Source: CAD feature listing. Evaluate the final solid. Frame: model axes, mm. A direction names the side the tool comes from. Give positions to 0.01 mm unless a question says otherwise; leave off trailing zeros. Order: outer loops, then holes, each group sorted by start corner. A loop starts at its lowest first (then second) coordinate and runs counter-clockwise, first axis right, second up. Notation, with made-up numbers: M -36.75,59.5 L 9.25,59.5 A11 cw 9.25,79.5 Z; hole C 12.25,3.5 d3. An arc over 180 degrees is marked long. Answer as a JSON object with one key per item and string values. Group by question number.
1. Pin query (flat end, axial travel): P1, Ø3, axis at y = -12.5, z = -70.5, coming from the -X side; P2, Ø2, axis at y = -6.5, z = -92.5, coming from the -X side; P3, Ø3, axis at x = -96.5, z = -151.5, coming from the -Y side; P4, Ø20.5, axis at x = -29.5, z = -95.5, coming from the +Y side. Return the tip coordinate at first contact, or that it passes through.
2. Section query D-D (z = -73.5). Output: boundary loops of the cut face in (x, y), plus the area to 3 significant figures.
3. Section query A-A (x = -30.5). Output: boundary loops of the cut face in (y, z).
4. Material intervals for L1, parallel to X at y = -12.75, z = -97; L2, parallel to Y at x = -33.5, z = -73.5; L3, parallel to Y at x = -93.5, z = -63, sorted ascending. Write a range as [from, to].
5. Set-up query: faces 5 (the flat face through (-36, 3, -221.069)), 6 (the flat face through (-36, -9, -118.199)), 7 (the flat face through (-97, 1.27, -136)), 8 (the flat face through (28, 0, -138)). Return all of +Z, -Z, +X, -X, +Y, -Y with unobstructed straight access to the full face (end or side cutting, diameter ignored); none if empty.
6. Section query C-C (y = -10). Output: boundary loops of the cut face in (x, z), plus the area to 3 significant figures.
7. Pull-direction query (X, two-part tool) for faces 1 (the cylindrical face through (-49.26, 1.86, -85)), 2 (the flat face through (-27, -20.32, -116)), 3 (the cylindrical face through (-49.26, -18.65, -85)), 4 (the flat face through (-99.356, 3, -138)); classes: +X half, -X half, draft (parallel to the pull), parting line (faces both ways), or undercut.
from build123d import *

# Parameters (mm, degrees)
F0_W     = 3.81
F0_H     = 167.64
F0_W_2   = 120.65
F1_DEPTH = 5.08
F0_H_2   = 3.81
F2_DEPTH = 1.27
F3_DEPTH = 1.27
F4_DEPTH = 1.27
F5_W     = 41.148
F5_H     = 6.35
F5_H_2   = 40.64
F5_R     = 19.05
F6_DEPTH = 19.05
F7_DEPTH = 15.748
F8_DEPTH = 6.35


with BuildPart() as f1:
    # F0 (on Front) → F1 (new body)
    with BuildSketch(Plane.XZ):
        with Locations((-97.4510958609, -137.2491913055)):
            Rectangle(F0_W, F0_H)
        with Locations((-35.2210958609, -137.2491913055)):
            Rectangle(F0_W_2, F0_H)
        with Locations((27.0089041391, -137.2491913055)):
            Rectangle(F0_W, F0_H)
    extrude(amount=-F1_DEPTH)

    # F0 (on Front) → F2 (join)
    with BuildSketch(Plane.XZ):
        with Locations((-35.2210958609, -222.9741913055)):
            Rectangle(F0_W_2, F0_H_2)
    extrude(amount=-F2_DEPTH)

    # F0 (on Front) → F3 (cut)
    with BuildSketch(Plane.XZ):
        with Locations((-97.4510958609, -137.2491913055)):
            Rectangle(F0_W, F0_H)
        with Locations((27.0089041391, -137.2491913055)):
            Rectangle(F0_W, F0_H)
    extrude(amount=-F3_DEPTH, mode=Mode.SUBTRACT)

    # F0 (on Front) → F4 (join)
    with BuildSketch(Plane.XZ):
        Polygon((-99.3560958609, -221.0691913055), (-99.3560958609, -53.4291913055), (-101.8960958609, -53.4291913055), (-101.8960958609, -224.8791913055), (-95.5460958609, -224.8791913055), (-95.5460958609, -221.0691913055), align=None)
        with Locations((-97.4510958609, -137.2491913055)):
            Rectangle(F0_W, F0_H)
        with Locations((-35.2210958609, -137.2491913055)):
            Rectangle(F0_W_2, F0_H)
        with Locations((-35.2210958609, -222.9741913055)):
            Rectangle(F0_W_2, F0_H_2)
        with Locations((27.0089041391, -137.2491913055)):
            Rectangle(F0_W, F0_H)
        Polygon((31.4539041391, -53.4291913055), (28.9139041391, -53.4291913055), (28.9139041391, -221.0691913055), (25.1039041391, -221.0691913055), (25.1039041391, -224.8791913055), (31.4539041391, -224.8791913055), align=None)
    extrude(amount=F4_DEPTH)

    # F5 (on face) → F6 (join)
    with BuildSketch(Plane.XZ.offset(1.27)):
        with BuildLine():
            Line((-14.6470958609, -71.2091913055), (-14.6470958609, -66.0530825267))
            ThreePointArc((-14.6470958609, -66.0530825267), (-35.2210958609, -59.9820848724), (-55.7950958609, -66.0530825267))
            Line((-55.7950958609, -66.0530825267), (-55.7950958609, -71.2091913055))
            Line((-55.7950958609, -71.2091913055), (-14.6470958609, -71.2091913055))
        make_face()
        with Locations((-35.2210958609, -74.3841913055)):
            Rectangle(F5_W, F5_H)
        with Locations((-35.2210958609, -97.8791913055)):
            Rectangle(F5_W, F5_H_2)
        with Locations((-35.2210958609, -97.8791913055)):
            Circle(F5_R, mode=Mode.SUBTRACT)
        with BuildLine():
            Line((-55.7950958609, -71.2091913055), (-55.7950958609, -66.0530825267))
            ThreePointArc((-55.7950958609, -66.0530825267), (-59.109615393, -68.4593117924), (-62.1450958609, -71.2091913055))
            Line((-62.1450958609, -71.2091913055), (-55.7950958609, -71.2091913055))
        make_face()
        with BuildLine():
            ThreePointArc((-62.1450958609, -71.2091913055), (-73.118202294, -97.8791913055), (-62.1450958609, -124.5491913055))
            Line((-62.1450958609, -124.5491913055), (-62.1450958609, -71.2091913055))
        make_face()
        with BuildLine():
            Line((-14.6470958609, -71.2091913055), (-8.2970958609, -71.2091913055))
            ThreePointArc((-8.2970958609, -71.2091913055), (-11.3325763288, -68.4593117924), (-14.6470958609, -66.0530825267))
            Line((-14.6470958609, -66.0530825267), (-14.6470958609, -71.2091913055))
        make_face()
        Polygon((-8.2970958609, -124.5491913055), (-8.2970958609, -71.2091913055), (-14.6470958609, -71.2091913055), (-14.6470958609, -77.5591913055), (-14.6470958609, -118.1991913055), (-55.7950958609, -118.1991913055), (-55.7950958609, -77.5591913055), (-55.7950958609, -71.2091913055), (-62.1450958609, -71.2091913055), (-62.1450958609, -124.5491913055), align=None)
        with BuildLine():
            ThreePointArc((-8.2970958609, -124.5491913055), (-0.1744671385, -112.298778373), (2.6760105722, -97.8791913055))
            ThreePointArc((2.6760105722, -97.8791913055), (-0.1744671385, -83.459604238), (-8.2970958609, -71.2091913055))
            Line((-8.2970958609, -71.2091913055), (-8.2970958609, -124.5491913055))
        make_face()
        with BuildLine():
            ThreePointArc((-62.1450958609, -124.5491913055), (-35.2210958609, -135.7762977386), (-8.2970958609, -124.5491913055))
            Line((-8.2970958609, -124.5491913055), (-62.1450958609, -124.5491913055))
        make_face()
        with BuildLine():
            ThreePointArc((-8.2970958609, -71.2091913055), (-0.1744671385, -83.459604238), (2.6760105722, -97.8791913055))
            ThreePointArc((2.6760105722, -97.8791913055), (-0.1744671385, -112.298778373), (-8.2970958609, -124.5491913055))
            ThreePointArc((-8.2970958609, -124.5491913055), (-35.2210958609, -135.7762977386), (-62.1450958609, -124.5491913055))
            ThreePointArc((-62.1450958609, -124.5491913055), (-73.118202294, -97.8791913055), (-62.1450958609, -71.2091913055))
            ThreePointArc((-62.1450958609, -71.2091913055), (-59.109615393, -68.4593117924), (-55.7950958609, -66.0530825267))
            Line((-55.7950958609, -66.0530825267), (-55.7950958609, -63.0672666147))
            ThreePointArc((-55.7950958609, -63.0672666147), (-55.2611376389, -133.0012114954), (5.2160105722, -97.8791913055))
            ThreePointArc((5.2160105722, -97.8791913055), (-0.099075671, -77.8391495275), (-14.6470958609, -63.0672666147))
            Line((-14.6470958609, -63.0672666147), (-14.6470958609, -66.0530825267))
            ThreePointArc((-14.6470958609, -66.0530825267), (-11.3325763288, -68.4593117924), (-8.2970958609, -71.2091913055))
        make_face()
    extrude(amount=F6_DEPTH)

    # F5 (on face) → F7 (cut)
    with BuildSketch(Plane.XZ.offset(1.27)):
        with Locations((-35.2210958609, -97.8791913055)):
            Rectangle(F5_W, F5_H_2)
        with Locations((-35.2210958609, -97.8791913055)):
            Circle(F5_R, mode=Mode.SUBTRACT)
        with Locations((-35.2210958609, -74.3841913055)):
            Rectangle(F5_W, F5_H)
        with BuildLine():
            Line((-14.6470958609, -71.2091913055), (-14.6470958609, -66.0530825267))
            ThreePointArc((-14.6470958609, -66.0530825267), (-35.2210958609, -59.9820848724), (-55.7950958609, -66.0530825267))
            Line((-55.7950958609, -66.0530825267), (-55.7950958609, -71.2091913055))
            Line((-55.7950958609, -71.2091913055), (-14.6470958609, -71.2091913055))
        make_face()
        with BuildLine():
            ThreePointArc((-55.7950958609, -66.0530825267), (-35.2210958609, -59.9820848724), (-14.6470958609, -66.0530825267))
            Line((-14.6470958609, -66.0530825267), (-14.6470958609, -63.0672666147))
            ThreePointArc((-14.6470958609, -63.0672666147), (-35.2210958609, -57.4420848724), (-55.7950958609, -63.0672666147))
            Line((-55.7950958609, -63.0672666147), (-55.7950958609, -66.0530825267))
        make_face()
        with BuildLine():
            ThreePointArc((-8.2970958609, -71.2091913055), (-0.1744671385, -83.459604238), (2.6760105722, -97.8791913055))
            ThreePointArc((2.6760105722, -97.8791913055), (-0.1744671385, -112.298778373), (-8.2970958609, -124.5491913055))
            ThreePointArc((-8.2970958609, -124.5491913055), (-35.2210958609, -135.7762977386), (-62.1450958609, -124.5491913055))
            ThreePointArc((-62.1450958609, -124.5491913055), (-73.118202294, -97.8791913055), (-62.1450958609, -71.2091913055))
            ThreePointArc((-62.1450958609, -71.2091913055), (-59.109615393, -68.4593117924), (-55.7950958609, -66.0530825267))
            Line((-55.7950958609, -66.0530825267), (-55.7950958609, -63.0672666147))
            ThreePointArc((-55.7950958609, -63.0672666147), (-55.2611376389, -133.0012114954), (5.2160105722, -97.8791913055))
            ThreePointArc((5.2160105722, -97.8791913055), (-0.099075671, -77.8391495275), (-14.6470958609, -63.0672666147))
            Line((-14.6470958609, -63.0672666147), (-14.6470958609, -66.0530825267))
            ThreePointArc((-14.6470958609, -66.0530825267), (-11.3325763288, -68.4593117924), (-8.2970958609, -71.2091913055))
        make_face()
    extrude(amount=F7_DEPTH, mode=Mode.SUBTRACT)

    # F5 (on face) → F8 (cut)
    with BuildSketch(Plane.XZ.offset(1.27)):
        with Locations((-35.2210958609, -97.8791913055)):
            Circle(F5_R)
    extrude(amount=-F8_DEPTH, mode=Mode.SUBTRACT)


solid = f1.part
Answer sheet:
{
 "1": {"P1": "x = -62.91", "P2": "x = -72.86", "P3": "y = -1.27", "P4": "through"},
 "2": {"outline": "M -101.9,-1.27 L -64.24,-1.27 L -64.24,-17.02 L -67.48,-17.02 L -67.48,-20.32 L -2.96,-20.32 L -2.96,-17.02 L -6.21,-17.02 L -6.21,-1.27 L 31.45,-1.27 L 31.45,0 L 25.1,0 L 25.1,1.27 L 28.91,1.27 L 28.91,5.08 L -99.36,5.08 L -99.36,1.27 L -95.55,1.27 L -95.55,0 L -101.9,0 Z; hole M -55.8,-17.02 L -14.65,-17.02 L -14.65,-1.27 L -55.8,-1.27 Z", "area": "1,290 mm^2"},
 "3": {"outline": "M -20.32,-138.04 L -17.02,-138.04 L -17.02,-135.48 L -1.27,-135.48 L -1.27,-224.88 L 1.27,-224.88 L 1.27,-221.07 L 5.08,-221.07 L 5.08,-116.33 L -1.27,-116.33 L -1.27,-118.2 L -17.02,-118.2 L -17.02,-116.33 L -20.32,-116.33 Z; M -20.32,-79.42 L -17.02,-79.42 L -17.02,-60.28 L -20.32,-60.28 Z; M -1.27,-79.42 L 5.08,-79.42 L 5.08,-53.43 L -1.27,-53.43 Z"},
 "4": {"L1": "[-73.11, -55.8], [-14.65, 2.67]", "L2": "[-20.32, -17.02], [-1.27, 5.08]", "L3": "[-1.27, 5.08]"},
 "5": {"face 5": "-Z, +X, -X, +Y", "face 6": "+Z", "face 7": "+Z, -Z, -X", "face 8": "+Z, -Z, +X"},
 "6": {"outline": "M -55.8,-118.2 L -55.8,-66.05 A37.9 ccw long -14.65,-66.05 L -14.65,-118.2 Z", "area": "2,200 mm^2"},
 "7": {"face 1": "undercut", "face 2": "draft", "face 3": "undercut", "face 4": "-X half"}
}
